Input: part model. Units: mm. Frame: model coordinates. A direction names the side the tool comes from. Round coordinates to 2 decimals unless told otherwise and drop trailing zeros. Order: outer loops, then holes, each group sorted by start corner. A loop starts at its lowest first (then second) coordinate and runs counter-clockwise, first axis right, second up. Notation, with made-up numbers: (30, 39.25) -> (52, 39.25) arc R21 ccw to (52, 45.25) -> close; hole circle Ø11 at (19, -1). An arc over 180 degrees is marked (long way). Answer as CSV lines item,"result". Start each with the question number.
1) First-contact query: P1, Ø0.6, axis at y = 8.5, z = 4, coming from the +X side; P2, Ø1.4, axis at y = 9.5, z = 2.5, coming from the +X side; P3, Ø3, axis at x = -8.5, z = 2.5, coming from the +Y side. Flat tips, straight axial feed; report the tip coordinate or a pass-through.
2) Section query C-C, the plane y = 5. State how many separate pieces and enclosed holes the cut face has, and give its area (3 significant figures).
3) Access query for faces 5 (the face through (28.195, 3.863, 2.965)), 6 (the face through (22, 9.59, 3.04)), 7 (the face through (27.24, 0.77, 5.26)), 8 (the face through (30.73, 3.757, 5.276)). Directions: +Z, -Z, +X, -X, +Y, -Y. A direction counts if a zero-diameter tool reaches every point of the face in a straight line with its end or side. Return the directions, or none.
4) Section query A-A, the plane y = 1. Output: boundary loops of the cut face in (x, z).
5) Section query B-B, the plane x = 4. Output: boundary loops of the cut face in (y, z), and give its area (3 significant figures).
6) Mould query, pull axis X, two halves, no side actions, for faces 1 (the face through (-27.2, 0.75, 0.78)), 2 (the face through (30.77, 3.757, 0.764)), 3 (the face through (-30.39, 9.71, 2.96)), 4 (the face through (1, 7, 6)). Classes: +X half, -X half, draft (parallel to the pull), parting line (faces both ways), or undercut.
7) Line query: L1, parallel to X at y = 5, z = 3; L2, parallel to X at y = 1.5, z = 3; L3, parallel to X at y = 3.25, z = 3. Output: solid intervals per line, ascending.
```python
from build123d import *

# Parameters (mm, degrees)
BOSS_EXTRUDE1_DEPTH   = 6
M2X0_4_TAPPED_HOLE1_D = 1.6
FILLET1_R             = 2.54
SKETCH4_W             = 9.9041
SKETCH4_H             = 2.536063356
CUT_EXTRUDE1_DEPTH    = 34.630699773
BOSS_EXTRUDE2_DEPTH   = 6
FILLET2_R             = 0.508


with BuildPart() as part:
    # Sketch1 → Boss-Extrude1 (new body)
    with BuildSketch(Plane.XY):
        with BuildLine():
            Line((-31.4941, 0), (-26.4941, 0))
            Line((-26.4941, 0), (-26.4941, 1.524))
            ThreePointArc((-26.4941, 1.524), (-25.750151224, 3.320051224), (-23.9541, 4.064))
            Line((-23.9541, 4.064), (23.9541, 4.064))
            ThreePointArc((23.9541, 4.064), (25.750151224, 3.320051224), (26.4941, 1.524))
            Line((26.4941, 1.524), (26.4941, 0))
            Line((26.4941, 0), (31.4941, 0))
            Line((31.4941, 0), (31.4941, 10.156063356))
            Line((31.4941, 10.156063356), (17.963402264, 10.156063356))
            Line((17.963402264, 10.156063356), (17.963402264, 8.886063356))
            ThreePointArc((17.963402264, 8.886063356), (18.668015075, 8.290353704), (18.034, 7.62))
            Line((18.034, 7.62), (-18.034, 7.62))
            ThreePointArc((-18.034, 7.62), (-18.668015075, 8.290353704), (-17.963402264, 8.886063356))
            Line((-17.963402264, 8.886063356), (-17.963402264, 10.156063356))
            Line((-17.963402264, 10.156063356), (-31.4941, 10.156063356))
            Line((-31.4941, 10.156063356), (-31.4941, 0))
        make_face()
    extrude(amount=BOSS_EXTRUDE1_DEPTH)

    # M2x0.4 Tapped Hole1 (through all)
    with Locations(Plane(origin=(0, 0, 0), x_dir=(-1, 0, 0), z_dir=(0, -1, 0))):
        with Locations((28.9941, -3), (-28.9941, -3)):
            Hole(M2X0_4_TAPPED_HOLE1_D / 2)

    # Fillet1
    # the kernel refuses this fillet: 2.54 mm, written as the material it takes off along each edge
    with BuildSketch(Plane(origin=(-26.4941, -6.35, 0), x_dir=(-1, 0, 0), z_dir=(0, 1, 0)), Plane(origin=(26.4941, 1.524, 0), x_dir=(1, 0, 0), z_dir=(0, -1, 0))) as fillet1_piece_1:
        with BuildLine():
            CenterArc((FILLET1_R, FILLET1_R), FILLET1_R, 180, 90)
            Line((0, FILLET1_R), (0, 0))
            Line((0, 0), (FILLET1_R, 0))
        make_face()
    extrude(amount=7.874, mode=Mode.SUBTRACT)
    with BuildSketch(Plane(origin=(-23.9541, 1.524, 0), x_dir=(-1, 0, 0), z_dir=(0, -1, 0))) as fillet1_piece_2:
        with BuildLine():
            CenterArc((2.54 + FILLET1_R, -FILLET1_R), FILLET1_R, 90, 90)
            Line((2.54, -FILLET1_R), (2.54, 0))
            Line((2.54, 0), (2.54 + FILLET1_R, 0))
        make_face()
    revolve(axis=Axis((-23.9541, 1.524, 0), (0, 0, -1)), revolution_arc=90, mode=Mode.SUBTRACT)
    with BuildSketch(Plane(origin=(23.9541, 1.524, 0), x_dir=(0, 1, 0), z_dir=(-1, 0, 0))) as fillet1_piece_3:
        with BuildLine():
            CenterArc((2.54 + FILLET1_R, -FILLET1_R), FILLET1_R, 90, 90)
            Line((2.54, -FILLET1_R), (2.54, 0))
            Line((2.54, 0), (2.54 + FILLET1_R, 0))
        make_face()
    revolve(axis=Axis((23.9541, 1.524, 0), (0, 0, -1)), revolution_arc=90, mode=Mode.SUBTRACT)
    with BuildSketch(Plane(origin=(-26.4941, -6.35, 6), x_dir=(-1, 0, 0), z_dir=(0, 1, 0)), Plane(origin=(26.4941, 1.524, 6), x_dir=(1, 0, 0), z_dir=(0, -1, 0))) as fillet1_piece_4:
        with BuildLine():
            CenterArc((FILLET1_R, -FILLET1_R), FILLET1_R, 90, 90)
            Line((0, -FILLET1_R), (0, 0))
            Line((0, 0), (FILLET1_R, 0))
        make_face()
    extrude(amount=7.874, mode=Mode.SUBTRACT)
    with BuildSketch(Plane(origin=(-23.9541, 1.524, 6), x_dir=(-1, 0, 0), z_dir=(0, -1, 0))) as fillet1_piece_5:
        with BuildLine():
            CenterArc((2.54 + FILLET1_R, FILLET1_R), FILLET1_R, 180, 90)
            Line((2.54, FILLET1_R), (2.54, 0))
            Line((2.54, 0), (2.54 + FILLET1_R, 0))
        make_face()
    revolve(axis=Axis((-23.9541, 1.524, 6), (0, 0, -1)), revolution_arc=90, mode=Mode.SUBTRACT)
    with BuildSketch(Plane(origin=(-23.9541, 4.064, 6), x_dir=(0, 1, 0), z_dir=(1, 0, 0))) as fillet1_piece_6:
        with BuildLine():
            CenterArc((FILLET1_R, -FILLET1_R), FILLET1_R, 90, 90)
            Line((0, -FILLET1_R), (0, 0))
            Line((0, 0), (FILLET1_R, 0))
        make_face()
    extrude(amount=47.9082, mode=Mode.SUBTRACT)
    with BuildSketch(Plane(origin=(23.9541, 1.524, 6), x_dir=(0, 1, 0), z_dir=(-1, 0, 0))) as fillet1_piece_7:
        with BuildLine():
            CenterArc((2.54 + FILLET1_R, FILLET1_R), FILLET1_R, 180, 90)
            Line((2.54, FILLET1_R), (2.54, 0))
            Line((2.54, 0), (2.54 + FILLET1_R, 0))
        make_face()
    revolve(axis=Axis((23.9541, 1.524, 6), (0, 0, -1)), revolution_arc=90, mode=Mode.SUBTRACT)
    with BuildSketch(Plane(origin=(-31.4941, 16.506063356, 0), x_dir=(1, 0, 0), z_dir=(0, -1, 0)), Plane(origin=(31.4941, -6.35, 0), x_dir=(-1, 0, 0), z_dir=(0, 1, 0))) as fillet1_piece_8:
        with BuildLine():
            CenterArc((FILLET1_R, FILLET1_R), FILLET1_R, 180, 90)
            Line((0, FILLET1_R), (0, 0))
            Line((0, 0), (FILLET1_R, 0))
        make_face()
    extrude(amount=22.856063356, mode=Mode.SUBTRACT)
    with BuildSketch(Plane(origin=(-31.4941, 16.506063356, 6), x_dir=(1, 0, 0), z_dir=(0, -1, 0)), Plane(origin=(31.4941, -6.35, 6), x_dir=(-1, 0, 0), z_dir=(0, 1, 0))) as fillet1_piece_9:
        with BuildLine():
            CenterArc((FILLET1_R, -FILLET1_R), FILLET1_R, 90, 90)
            Line((0, -FILLET1_R), (0, 0))
            Line((0, 0), (FILLET1_R, 0))
        make_face()
    extrude(amount=22.856063356, mode=Mode.SUBTRACT)
    with BuildSketch(Plane(origin=(-23.9541, 4.064, 0), x_dir=(0, 1, 0), z_dir=(1, 0, 0))) as fillet1_piece_10:
        with BuildLine():
            CenterArc((FILLET1_R, FILLET1_R), FILLET1_R, 180, 90)
            Line((0, FILLET1_R), (0, 0))
            Line((0, 0), (FILLET1_R, 0))
        make_face()
    extrude(amount=47.9082, mode=Mode.SUBTRACT)
    with BuildSketch(Plane(origin=(31.4941, 10.156063356, -6.35), x_dir=(0, -1, 0), z_dir=(0, 0, 1)), Plane(origin=(-31.4941, 10.156063356, -6.35), x_dir=(1, 0, 0), z_dir=(0, 0, 1))) as fillet1_piece_11:
        with BuildLine():
            CenterArc((FILLET1_R, -FILLET1_R), FILLET1_R, 90, 90)
            Line((0, -FILLET1_R), (0, 0))
            Line((0, 0), (FILLET1_R, 0))
        make_face()
    extrude(amount=18.7, mode=Mode.SUBTRACT)

    # Sketch4 → Cut-Extrude1 (cut, through all)
    with BuildSketch(Plane.XY.offset(6)):
        with Locations((26.54205, 8.888031678)):
            Rectangle(SKETCH4_W, SKETCH4_H)
    extrude(amount=-CUT_EXTRUDE1_DEPTH, mode=Mode.SUBTRACT)

    # Sketch5 → Boss-Extrude2 (add)
    with BuildSketch(Plane.XY.offset(6)):
        with BuildLine():
            Line((22.781680466, 9.873540862), (30.033107734, 9.873540862))
            ThreePointArc((30.033107734, 9.873540862), (30.500081052, 10.066967543), (30.693507734, 10.533940862))
            Line((30.693507734, 10.533940862), (30.693507734, 11.143540862))
            ThreePointArc((30.693507734, 11.143540862), (30.414801602, 11.937415201), (29.701009362, 12.382852302))
            ThreePointArc((29.701009362, 12.382852302), (29.338161991, 12.065038452), (29.004680466, 12.413540862))
            Line((29.004680466, 12.413540862), (28.813361866, 12.413540862))
            ThreePointArc((28.813361866, 12.413540862), (28.464521166, 12.064700162), (28.115680466, 12.413540862))
            Line((28.115680466, 12.413540862), (27.924361866, 12.413540862))
            ThreePointArc((27.924361866, 12.413540862), (27.575521166, 12.064700162), (27.226680466, 12.413540862))
            Line((27.226680466, 12.413540862), (27.035361866, 12.413540862))
            ThreePointArc((27.035361866, 12.413540862), (26.686521166, 12.064700162), (26.337680466, 12.413540862))
            Line((26.337680466, 12.413540862), (26.146361866, 12.413540862))
            ThreePointArc((26.146361866, 12.413540862), (25.797521166, 12.064700162), (25.448680466, 12.413540862))
            Line((25.448680466, 12.413540862), (25.257361866, 12.413540862))
            ThreePointArc((25.257361866, 12.413540862), (24.908521166, 12.064700162), (24.559680466, 12.413540862))
            Line((24.559680466, 12.413540862), (24.368361866, 12.413540862))
            ThreePointArc((24.368361866, 12.413540862), (24.019521166, 12.064700162), (23.670680466, 12.413540862))
            Line((23.670680466, 12.413540862), (23.479361866, 12.413540862))
            ThreePointArc((23.479361866, 12.413540862), (23.130521166, 12.064700162), (22.781680466, 12.413540862))
            Line((22.781680466, 12.413540862), (19.233402264, 12.413540862))
            ThreePointArc((19.233402264, 12.413540862), (18.335376652, 12.041566474), (17.963402264, 11.143540862))
            Line((17.963402264, 11.143540862), (17.963402264, 10.156063356))
            Line((17.963402264, 10.156063356), (21.59, 10.156063356))
            Line((21.59, 10.156063356), (21.59, 8.888031678))
            ThreePointArc((21.59, 8.888031678), (22.008484067, 9.595245842), (22.781680466, 9.873540862))
        make_face()
    extrude(amount=-BOSS_EXTRUDE2_DEPTH)

    # Fillet2
    fillet2_edges = [part.edges().sort_by_distance(p)[0] for p in [
        (21.59, 7.62, 3),
    ]]
    fillet(fillet2_edges, radius=FILLET2_R)


solid = part.part
```
Findings:
1,P1,"stops at x = 21.59"
1,P2,"stops at x = 30.6"
1,P3,"stops at y = 7.62"
2,separate pieces,"1"
2,enclosed holes,"2"
2,area,"310 mm^2"
3,face 5,"-Y"
3,face 6,"+Z, -Z, +X"
3,face 7,"+Z, -Y"
3,face 8,"+Z, +X, -Y"
4,outline,"(-31.49, 2.54) arc R2.54 ccw to (-28.99, 0) arc R2.54 ccw to (-26.49, 2.54) -> (-26.49, 3.46) arc R2.54 ccw to (-28.99, 6) arc R2.54 ccw to (-31.49, 3.46) -> close; (26.49, 2.54) arc R2.54 ccw to (28.99, 0) arc R2.54 ccw to (31.49, 2.54) -> (31.49, 3.46) arc R2.54 ccw to (28.99, 6) arc R2.54 ccw to (26.49, 3.46) -> close; hole circle Ø1.6 at (-28.99, 3); hole circle Ø1.6 at (28.99, 3)"
5,outline,"(4.06, 2.54) arc R2.54 ccw to (6.6, 0) -> (7.62, 0) -> (7.62, 6) -> (6.6, 6) arc R2.54 ccw to (4.06, 3.46) -> close"
5,area,"18.6 mm^2"
6,face 1,"undercut"
6,face 2,"+X half"
6,face 3,"-X half"
6,face 4,"draft"
7,L1,"x = -31.49 to -29.79, -28.19 to 28.19, 29.79 to 31.49"
7,L2,"x = -31.49 to -29.79, -28.19 to -26.49, 26.49 to 28.19, 29.79 to 31.49"
7,L3,"x = -31.49 to -29.79, -28.19 to -25.82, 25.82 to 28.19, 29.79 to 31.49"
